Can you work these out from the model? Positions are in its coordinate system, mm. A direction names the side the tool comes from. Give positions to 0.01 mm unless a question says otherwise; leave off trailing zeros. Order: outer loops, then holes, each group sorted by start corner. A loop starts at its lowest first (then second) coordinate and runs counter-clockwise, first axis right, second up. Notation, with made-up numbers: (-31, 21) - (-1, 21) arc R25 ccw to (-1, 33) - close; hole circle Ø9 at (74.5, 54.5). An arc over 180 degrees is marked (long way). Answer as a JSON object with one key per item and string values.
```python
from build123d import *

# Parameters (mm, degrees)
BOSS_EXTRUDE1_DEPTH = 3.5
BOSS_EXTRUDE4_DEPTH = 7
SKETCH3_R           = 26
SKETCH3_R_2         = 4.2
SKETCH3_R_3         = 5.95
CUT_EXTRUDE1_DEPTH  = 156.479666598
CUT_EXTRUDE3_DEPTH  = 156.479666598
CUT_EXTRUDE5_DEPTH  = 156.479666598
CUT_EXTRUDE6_DEPTH  = 156.479666598
CIRPATTERN1_COUNT   = 6


with BuildPart() as part:
    # Sketch2 → Boss-Extrude1 (new, symmetric)
    with BuildSketch(Plane.XY):
        with BuildLine():
            Line((-45.478900867, 6.904315749), (-63.304842767, -110.515610278))
            ThreePointArc((-63.304842767, -110.515610278), (-57.554578813, -119.77853103), (-47.500804036, -115.560848118))
            Line((-47.500804036, -115.560848118), (-26.78284273, -74.506517319))
            ThreePointArc((-26.78284273, -74.506517319), (-6.255979799, -58.681947165), (18.940409864, -64.757395322))
            Line((18.940409864, -64.757395322), (84.696685238, -118.290602278))
            ThreePointArc((84.696685238, -118.290602278), (95.084548335, -118.462755244), (97.694455028, -108.406626595))
            Line((97.694455028, -108.406626595), (42.136301343, 18.453512109))
            ThreePointArc((42.136301343, 18.453512109), (-6.011591057, 45.605490601), (-45.478900867, 6.904315749))
        make_face()
    extrude(amount=BOSS_EXTRUDE1_DEPTH, both=True)

    # Sketch4 → Boss-Extrude4 (add, through all)
    with BuildSketch(Plane.XY.offset(3.5)):
        with BuildLine():
            Line((29.393386496, 35.38401942), (44.963587603, 19.409766638))
            ThreePointArc((44.963587603, 19.409766638), (46.631084985, 17.126299569), (47.592760093, 14.467361743))
            Line((47.592760093, 14.467361743), (50.74066814, -0.658267229))
            ThreePointArc((50.74066814, -0.658267229), (51.004474494, -1.661692304), (51.370828532, -2.632382983))
            Line((51.370828532, -2.632382983), (97.694455028, -108.406626595))
            ThreePointArc((97.694455028, -108.406626595), (95.084548335, -118.462755244), (84.696685238, -118.290602278))
            Line((84.696685238, -118.290602278), (18.940409864, -64.757395322))
            ThreePointArc((18.940409864, -64.757395322), (-6.255979799, -58.681947165), (-26.78284273, -74.506517319))
            Line((-26.78284273, -74.506517319), (-47.500804036, -115.560848118))
            ThreePointArc((-47.500804036, -115.560848118), (-57.554578813, -119.77853103), (-63.304842767, -110.515610278))
            Line((-63.304842767, -110.515610278), (-45.478900867, 6.904315749))
            ThreePointArc((-45.478900867, 6.904315749), (-16.354183668, 42.994658698), (29.393386496, 35.38401942))
        make_face()
    extrude(amount=-BOSS_EXTRUDE4_DEPTH)

    # Sketch3 → Cut-Extrude1 (cut, through all)
    with BuildSketch(Plane(origin=(0, 0, -3.5), x_dir=(-1, 0, 0), z_dir=(0, 0, -1))):
        Circle(SKETCH3_R)
        with Locations((19.5, 33.774990748)):
            Circle(SKETCH3_R_2)
        with Locations((-19.5, 33.774990748)):
            Circle(SKETCH3_R_2)
        with Locations((-36.7, 13.4)):
            Circle(SKETCH3_R_3)
        with Locations((-39, 0)):
            Circle(SKETCH3_R_2)
        with Locations((-36.7, -13.4)):
            Circle(SKETCH3_R_3)
        with Locations((-19.5, -33.774990748)):
            Circle(SKETCH3_R_2)
        with Locations((19.5, -33.774990748)):
            Circle(SKETCH3_R_2)
        with Locations((39, 0)):
            Circle(SKETCH3_R_2)
        with Locations((-90, -111.776398371)):
            Circle(SKETCH3_R_2)
        with Locations((55, -111.776398371)):
            Circle(SKETCH3_R_2)
    extrude(amount=-CUT_EXTRUDE1_DEPTH, mode=Mode.SUBTRACT)

    # Sketch5 → Cut-Extrude3 (cut, through all)
    with BuildSketch(Plane(origin=(0, 0, -3.5), x_dir=(-1, 0, 0), z_dir=(0, 0, -1))):
        with BuildLine():
            Line((-50.350110091, -31.309459743), (-20.150300754, -47.836521791))
            ThreePointArc((-20.150300754, -47.836521791), (-17.571466955, -51.766920177), (-19.393917714, -56.100173974))
            Line((-19.393917714, -56.100173974), (-74.370376325, -100.857364368))
            ThreePointArc((-74.370376325, -100.857364368), (-81.790278537, -100.980330772), (-83.654497603, -93.797381737))
            Line((-83.654497603, -93.797381737), (-57.330494783, -33.689793067))
            ThreePointArc((-57.330494783, -33.689793067), (-54.364230538, -30.963194657), (-50.350110091, -31.309459743))
        make_face()
    extrude(amount=-CUT_EXTRUDE3_DEPTH, mode=Mode.SUBTRACT)

    # Sketch7 → Cut-Extrude5 (cut, through all)
    with BuildSketch(Plane(origin=(0, 0, -3.5), x_dir=(-1, 0, 0), z_dir=(0, 0, -1))):
        with BuildLine():
            Line((23.433420065, -41.81343059), (37.676807322, -33.666002693))
            ThreePointArc((37.676807322, -33.666002693), (42.335474705, -33.504479598), (45.102778478, -37.255652924))
            Line((45.102778478, -37.255652924), (53.940298501, -95.468618789))
            ThreePointArc((53.940298501, -95.468618789), (51.202077571, -99.879533433), (46.414565772, -97.871112999))
            Line((46.414565772, -97.871112999), (21.45222531, -48.406198584))
            ThreePointArc((21.45222531, -48.406198584), (21.12757408, -44.71456882), (23.433420065, -41.81343059))
        make_face()
    extrude(amount=-CUT_EXTRUDE5_DEPTH, mode=Mode.SUBTRACT)

    # Sketch8 → Cut-Extrude6 (cut, through all)
    with BuildSketch(Plane(origin=(0, 0, -3.5), x_dir=(-1, 0, 0), z_dir=(0, 0, -1))):
        with BuildLine():
            ThreePointArc((7.583333333, 41.309721078), (0, 42), (-7.583333333, 41.309721078))
            ThreePointArc((-7.583333333, 41.309721078), (-12.401388725, 34.324999019), (-5.416666667, 29.506943627))
            ThreePointArc((-5.416666667, 29.506943627), (0, 30), (5.416666667, 29.506943627))
            ThreePointArc((5.416666667, 29.506943627), (12.401388725, 34.324999019), (7.583333333, 41.309721078))
        make_face()
    cut_extrude6 = extrude(amount=-CUT_EXTRUDE6_DEPTH, mode=Mode.SUBTRACT)

    # CirPattern1: Cut-Extrude6 ×6 about axis, 2 skipped
    cirpattern1_axis = Axis((0, 0, 37.050489462), (0, 0, -1))
    add([cut_extrude6.rotate(cirpattern1_axis, i * 360 / CIRPATTERN1_COUNT) for i in range(1, CIRPATTERN1_COUNT) if i not in (1, 2)], mode=Mode.SUBTRACT)


solid = part.part
```
Q1. Which directions (+Z, -Z, +X, -X, +Y, -Y) give clear straight access to the entire face, cutting with the end or side of a thin tool? Please do faces 1 (the face through (40.48, 24.01, 0.05)), 2 (the face through (-42.274, -33.475, -0.049)).
Recorded:
{"face 1": "+Z, -Z, +X, +Y", "face 2": "+Z, -Z"}
Q2. I need wall thicknesses on L1, parallel to Y at x = -19.5, z = 0 (3 decimals); L2, parallel to Y at x = 19.5, z = 1.75 (3 decimals); L3, parallel to Y at x = -1.5, z = -0.5. Which ranges of each line are inside material? Lowest first, please.
Recorded:
{"L1": "y = -65.224 to -37.975, -29.575 to -17.197, 17.197 to 29.575, 37.975 to 41.662", "L2": "y = -65.213 to -56.187, -48.261 to -37.975, -29.575 to -17.197, 17.197 to 29.575, 37.975 to 41.662", "L3": "y = -58.06 to -41.97, -29.96 to -25.96, 25.96 to 29.96, 41.97 to 45.98"}
Q3. I'm going to push flat-ended pins straight in: pin 1 Ø9.5 at (x, y) = (-19.5, 33.77) entering from -Z; pin 2 Ø3 at (x, z) = (10.5, 2) entering from +Y; pin 3 Ø4 at (y, z) = (-1.5, 2) entering from +X; pin 4 Ø2 at (y, z) = (-74, -1.5) entering from +X. Where does each tip first touch, or does it pass through?
Recorded:
{"pin 1": "stops at z = -3.5", "pin 2": "stops at y = 45.11", "pin 3": "stops at x = 51.75", "pin 4": "stops at x = 83.06"}
Q4. If we section it at A-A, the plane x = 0: Please give me the cut outline in (y, z).
Recorded:
{"outline": "(-58.02, -3.5) - (-42, -3.5) - (-42, 3.5) - (-58.02, 3.5) - close; (-30, -3.5) - (-26, -3.5) - (-26, 3.5) - (-30, 3.5) - close; (26, -3.5) - (30, -3.5) - (30, 3.5) - (26, 3.5) - close; (42, -3.5) - (46, -3.5) - (46, 3.5) - (42, 3.5) - close"}
Q5. If we section it at D-D, the plane y = -70: Please give me the cut outline in (x, z), then the cut area to 3 significant figures.
Recorded:
{"outline": "(-57.15, -3.5) - (-50.07, -3.5) - (-50.07, 3.5) - (-57.15, 3.5) - close; (-32.35, -3.5) - (-23.98, -3.5) - (-23.98, 3.5) - (-32.35, 3.5) - close; (25.38, -3.5) - (36.47, -3.5) - (36.47, 3.5) - (25.38, 3.5) - close; (73.23, -3.5) - (80.87, -3.5) - (80.87, 3.5) - (73.23, 3.5) - close", "area": "239 mm^2"}
Q6. If we section it at C-C, the plane x = 90: Please give me the cut outline in (y, z).
Recorded:
{"outline": "(-120.18, -3.5) - (-115.98, -3.5) - (-115.98, 3.5) - (-120.18, 3.5) - close; (-107.58, -3.5) - (-90.84, -3.5) - (-90.84, 3.5) - (-107.58, 3.5) - close"}
Q7. We'd pull the mould along Y, two halves only. Please class faces 3 (the face through (-54.267, -50.984, 0.049)), 4 (the face through (-37.287, -95.321, 0.049)), 5 (the face through (-12.424, -34.455, -0.049)): released by +Y, released by -Y, zero draft, split by the parting line, or undercut.
Recorded:
{"face 3": "released by +Y", "face 4": "released by -Y", "face 5": "undercut"}
Q8. If we section it at B-B, the plane y = -105: Please give me the cut outline in (x, z).
Recorded:
{"outline": "(-62.47, -3.5) - (-42.17, -3.5) - (-42.17, 3.5) - (-62.47, 3.5) - close; (68.37, -3.5) - (96.2, -3.5) - (96.2, 3.5) - (68.37, 3.5) - close"}
